from build123d import *

# Parameters (mm, degrees)
SKETCH_1_W          = 96
SKETCH_1_H          = 20
EXTRUDE_1_DEPTH     = 10
SKETCH_2_R          = 5
CUT_EXTRUDE_1_DEPTH = 5
FILLET_1_R          = 10
SKETCH_3_R          = 3.1
CUT_EXTRUDE_2_DEPTH = 5
CHAMFER_1_SIZE      = 1
SKETCH_4_W          = 60
SKETCH_4_H          = 20
EXTRUDE_2_DEPTH     = 80
CUT_EXTRUDE_4_REACH = 105.942
SKETCH_6_R          = 1.1
CUT_EXTRUDE_5_DEPTH = 11
SKETCH_8_W          = 60
SKETCH_8_H          = 102
CUT_EXTRUDE_6_DEPTH = 12
SKETCH_9_R          = 1.1
CUT_EXTRUDE_7_DEPTH = 10
FILLET_8_R          = 7
SKETCH_10_W         = 12
SKETCH_10_H         = 10
EXTRUDE_3_DEPTH     = 60
FILLET_11_R         = 3
CHAMFER_4_SIZE      = 1


with BuildPart() as part:
    # 草图1 → 凸台-拉伸1 (new body)
    with BuildSketch(Plane(origin=(0, 0, 0), x_dir=(1, 0, 0), z_dir=(0, 1, 0))):
        Rectangle(SKETCH_1_W, SKETCH_1_H)
    extrude(amount=EXTRUDE_1_DEPTH)

    # 草图2 → 切除-拉伸1 (cut)
    with BuildSketch(Plane(origin=(0, 10, 0), x_dir=(1, 0, 0), z_dir=(0, 1, 0))):
        with Locations(Location((-38, 0, 0), (0, 0, 270))):
            Circle(SKETCH_2_R)
        with Locations(Location((38, 0, 0), (0, 0, 90))):
            Circle(SKETCH_2_R)
    extrude(amount=-CUT_EXTRUDE_1_DEPTH, mode=Mode.SUBTRACT)

    # 圆角1
    fillet_1_edges = [part.edges().sort_by_distance(p)[0] for p in [
        (48, 5, -10),
        (48, 5, 10),
        (-48, 5, 10),
        (-48, 5, -10),
    ]]
    fillet(fillet_1_edges, radius=FILLET_1_R - 0.0001)  # a hair under: the kernel refuses the full size

    # 草图3 → 切除-拉伸2 (cut)
    with BuildSketch(Plane(origin=(0, 5, 0), x_dir=(1, 0, 0), z_dir=(0, 1, 0))):
        with Locations(Location((-38, 0, 0), (0, 0, 270))):
            Circle(SKETCH_3_R)
        with Locations(Location((38, 0, 0), (0, 0, 270))):
            Circle(SKETCH_3_R)
    extrude(amount=-CUT_EXTRUDE_2_DEPTH, mode=Mode.SUBTRACT)

    # 倒角1
    chamfer_1_edges = [part.edges().sort_by_distance(p)[0] for p in [
        (-38, 0, -3.1),
        (38, 0, -3.1),
    ]]
    chamfer(chamfer_1_edges, length=CHAMFER_1_SIZE)

    # 草图4 → 凸台-拉伸2 (add)
    with BuildSketch(Plane(origin=(0, 10, 0), x_dir=(1, 0, 0), z_dir=(0, 1, 0))):
        Rectangle(SKETCH_4_W, SKETCH_4_H)
    extrude(amount=EXTRUDE_2_DEPTH)

    # 草图6 → 切除-拉伸4 (cut, up to next)
    with BuildSketch(Plane.XY.offset(10), mode=Mode.PRIVATE) as cut_extrude_4_sk1:
        with Locations((-9, 41)):
            Circle(SKETCH_6_R)
    cut_extrude_4_tool1 = extrude(cut_extrude_4_sk1.sketch, amount=-CUT_EXTRUDE_4_REACH, mode=Mode.PRIVATE) & part.part
    # 草图6 → 切除-拉伸4 (cut, up to next)
    with BuildSketch(Plane.XY.offset(10), mode=Mode.PRIVATE) as cut_extrude_4_sk2:
        with Locations((9, 41)):
            Circle(SKETCH_6_R)
    cut_extrude_4_tool2 = extrude(cut_extrude_4_sk2.sketch, amount=-CUT_EXTRUDE_4_REACH, mode=Mode.PRIVATE) & part.part
    # 草图6 → 切除-拉伸4 (cut, up to next)
    with BuildSketch(Plane.XY.offset(10), mode=Mode.PRIVATE) as cut_extrude_4_sk3:
        with Locations((9, 30)):
            Circle(SKETCH_6_R)
    cut_extrude_4_tool3 = extrude(cut_extrude_4_sk3.sketch, amount=-CUT_EXTRUDE_4_REACH, mode=Mode.PRIVATE) & part.part
    # 草图6 → 切除-拉伸4 (cut, up to next)
    with BuildSketch(Plane.XY.offset(10), mode=Mode.PRIVATE) as cut_extrude_4_sk4:
        with Locations((-9, 30)):
            Circle(SKETCH_6_R)
    cut_extrude_4_tool4 = extrude(cut_extrude_4_sk4.sketch, amount=-CUT_EXTRUDE_4_REACH, mode=Mode.PRIVATE) & part.part
    add(cut_extrude_4_tool1.solids().sort_by_distance((-9, 41, 10))[0], mode=Mode.SUBTRACT)
    add(cut_extrude_4_tool2.solids().sort_by_distance((9, 41, 10))[0], mode=Mode.SUBTRACT)
    add(cut_extrude_4_tool3.solids().sort_by_distance((9, 30, 10))[0], mode=Mode.SUBTRACT)
    add(cut_extrude_4_tool4.solids().sort_by_distance((-9, 30, 10))[0], mode=Mode.SUBTRACT)

    # 草图6<8> → 切除-拉伸5 (cut)
    with BuildSketch(Plane.XY.offset(10)):
        Polygon((0, 55), (11, 55), (11, 51.5), (-11, 51.5), (-11, 55), align=None)
    extrude(amount=-CUT_EXTRUDE_5_DEPTH, mode=Mode.SUBTRACT)

    # 草图8 → 切除-拉伸6 (cut)
    with BuildSketch(Plane(origin=(0, 0, -10), x_dir=(-1, 0, 0), z_dir=(0, 0, -1))):
        with Locations((0, 39)):
            Rectangle(SKETCH_8_W, SKETCH_8_H)
    extrude(amount=-CUT_EXTRUDE_6_DEPTH, mode=Mode.SUBTRACT)

    # 草图9 → 切除-拉伸7 (cut)
    with BuildSketch(Plane(origin=(0, 0, 2), x_dir=(-1, 0, 0), z_dir=(0, 0, -1))):
        with Locations((-22.5, 82.797945994)):
            Circle(SKETCH_9_R)
        with Locations((22.5, 82.797945994)):
            Circle(SKETCH_9_R)
        with Locations((22.5, 17.797945994)):
            Circle(SKETCH_9_R)
        with Locations((-22.5, 17.797945994)):
            Circle(SKETCH_9_R)
    extrude(amount=-CUT_EXTRUDE_7_DEPTH, mode=Mode.SUBTRACT)

    # 圆角8
    fillet_8_edges = [part.edges().sort_by_distance(p)[0] for p in [
        (-30, 90, 6),
        (30, 90, 6),
    ]]
    fillet(fillet_8_edges, radius=FILLET_8_R)

    # 草图10 → 凸台-拉伸3 (add)
    with BuildSketch(Plane.ZY.offset(-30)):
        with Locations((-4, 5)):
            Rectangle(SKETCH_10_W, SKETCH_10_H)
    extrude(amount=EXTRUDE_3_DEPTH)

    # 圆角11
    fillet_11_edges = [part.edges().sort_by_distance(p)[0] for p in [
        (-30, 10, 6),
        (30, 10, 6),
    ]]
    fillet(fillet_11_edges, radius=FILLET_11_R)

    # 倒角4
    chamfer_4_edges = [part.edges().sort_by_distance(p)[0] for p in [
        (0, 90, 2),
        (0, 90, 10),
        (30, 48, 10),
        (-30, 48, 10),
        (27.949747468, 87.949747468, 10),
        (-27.949747468, 87.949747468, 10),
        (30, 48, 2),
        (27.949747468, 87.949747468, 2),
        (-27.949747468, 87.949747468, 2),
        (-30, 48, 2),
        (35.50005, 10, 10),
        (-30.878679656, 10.878679656, 10),
        (-30.878679656, 10.878679656, 2),
        (30.878679656, 10.878679656, 2),
        (30.878679656, 10.878679656, 10),
        (0, 10, -10),
        (-35.50005, 10, 10),
        (-45.071097101, 10, -7.071097101),
        (-45.071097101, 10, 7.071097101),
        (45.071097101, 10, 7.071097101),
        (45.071097101, 10, -7.071097101),
    ]]
    chamfer(chamfer_4_edges, length=CHAMFER_4_SIZE)


solid = part.part
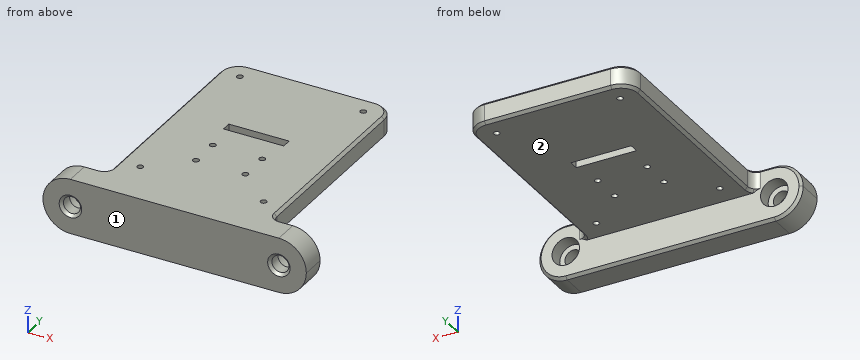
Geometry check sheet. Reference: the model listing, model coordinates, mm. Face numbers are marked on the shaded views. A direction names the side the tool comes from. Round coordinates to 2 decimals unless told otherwise and drop trailing zeros. Write each loop counter-clockwise with the first axis right and the second up, starting at its lowest first coordinate (ties: lowest second). Pieces come first, ordered by that corner, then holes.
Item 1: Access from +Z, -Z, +X, -X, +Y, -Y to the whole of each face (thin tool, end or side, straight path). Record for the marked faces 1 and 2.
Determined:
face 1: +Z, -Z, +X, -X, -Y
face 2: -Z, +X, -X, +Y
Item 2: Go/stop test with flat-tipped pins: pin 1 Ø4 at (x, y) = (-29, 66) entering from -Z; pin 2 Ø6 at (x, z) = (-25.5, 0.5) entering from +Y; pin 3 Ø1 at (x, z) = (-2, -8) entering from +Y; pin 4 Ø2 at (x, y) = (-9, 41) entering from +Z. Record where each tip stops, or that it passes through.
Determined:
pin 1: stops at z = 2
pin 2: stops at y = 89.95
pin 3: stops at y = 10
pin 4: passes through
Item 3: Material ranges on line 1 along Y through (x, z) = (-22.5, 5.25); line 2 along X through (y, z) = (7.5, 0); line 3 along Y through (x, z) = (22, 7), recorded low to high.
Determined:
line 1: y = 0 to 16.7, 18.9 to 81.7, 83.9 to 90
line 2: x = -48 to -43, -33 to 33, 43 to 48
line 3: y = 0 to 16.82, 18.78 to 81.82, 83.78 to 90
Item 4: Section check A-A (y = 41). Record the boundary of the cut face in (x, z).
Determined:
outline: (-30, 3) - (-29, 2) - (-10.1, 2) - (-10.1, 10) - (-29, 10) - (-30, 9) - close; (-7.9, 2) - (7.9, 2) - (7.9, 10) - (-7.9, 10) - close; (10.1, 2) - (29, 2) - (30, 3) - (30, 9) - (29, 10) - (10.1, 10) - close
Item 5: Section check B-B (x = 19). Record the boundary of the cut face in (y, z).
Determined:
outline: (0, -10) - (9, -10) - (10, -9) - (10, 2) - (89, 2) - (90, 3) - (90, 9) - (89, 10) - (0, 10) - close
